Design review of the part built by this model. Coordinates are the model's own, in mm. Round coordinates to 2 decimals unless told otherwise and drop trailing zeros. Write each loop counter-clockwise with the first axis right and the second up, starting at its lowest first coordinate (ties: lowest second). Pieces come first, ordered by that corner, then holes. Notation, with made-up numbers: (26.5, 57) - (31.5, 57) arc R32 cw to (31.5, 84) - close; hole circle Ø8 at (47.5, 49). An arc over 180 degrees is marked (long way). Use one line per item in the form item = value.
```python
from build123d import *

# Parameters (mm, degrees)
F1_DEPTH = 1.5
F2_R     = 42.5
F3_DEPTH = 1.501
F4_R     = 10
F5_R     = 20
F7_D     = 6


with BuildPart() as f1:
    # F0 (on Top) → F1 (new body)
    with BuildSketch(Plane.XY):
        with BuildLine():
            Line((0, 36.5856099731), (0, 196.5856099731))
            ThreePointArc((0, 196.5856099731), (-307.3351576975, 315.2560594706), (-635, 349.5099039223))
            Line((-635, 349.5099039223), (-621.0269461922, 189.7971680702))
            Line((-621.0269461922, 189.7971680702), (-361.6779078132, 171.4103170113))
            Line((-361.6779078132, 171.4103170113), (-225.8692382849, 137.4102393502))
            Line((-225.8692382849, 137.4102393502), (0, 36.5856099731))
        make_face()
    extrude(amount=F1_DEPTH)

    # F2 (on face) → F3 (cut, through all)
    with BuildSketch(Plane.XY.offset(1.5)):
        with Locations((-275.0559937421, 229.17509395)):
            Circle(F2_R)
        with Locations((-165, 190)):
            Circle(F2_R)
        with Locations((-65, 145)):
            Circle(F2_R)
    extrude(amount=-F3_DEPTH, mode=Mode.SUBTRACT)

    # F4
    f4_edges = [f1.edges().sort_by_distance(p)[0] for p in [
        (0, 196.58561, 0.75),
        (-635, 349.509904, 0.75),
        (-621.026946, 189.797168, 0.75),
        (0, 36.58561, 0.75),
    ]]
    fillet(f4_edges, radius=F4_R)

    # F5
    f5_edges = [f1.edges().sort_by_distance(p)[0] for p in [
        (-361.677908, 171.410317, 0.75),
        (-225.869238, 137.410239, 0.75),
    ]]
    fillet(f5_edges, radius=F5_R)

    # F7 (through all)
    with Locations(Plane.XY.offset(1.5)):
        with Locations((-624.1092854766, 339.7655997622), (-611.8086529213, 199.1687262985), (-411.8395238612, 325.6409079413), (-374.0631195885, 182.3134808013), (-205.1081070963, 275.4405101573), (-209.8076952351, 141.1916790514), (-10, 190.6420127613), (-10, 52.0005303507)):
            Hole(F7_D / 2)


solid = f1.part
```
Q1. We need section A-A on y = 125. Write out the cut boundary in (x, z).
Calculated:
outline = (-198.07, 0) - (-102.5, 0) - (-102.5, 1.5) - (-198.07, 1.5) - close; (-27.5, 0) - (0, 0) - (0, 1.5) - (-27.5, 1.5) - close
Q2. We need section D-D on x = -542. Write out the cut boundary in (y, z).
Calculated:
outline = (184.19, 0) - (348.65, 0) - (348.65, 1.5) - (184.19, 1.5) - close
Q3. We need section B-B on x = -170.5. Write out the cut boundary in (y, z), then the cut area to 3 significant figures.
Calculated:
outline = (112.69, 0) - (147.86, 0) - (147.86, 1.5) - (112.69, 1.5) - close; (232.14, 0) - (273.9, 0) - (273.9, 1.5) - (232.14, 1.5) - close
area = 115 mm2
Q4. To check wall thickness, follow line 1 along X through (y, z) = (200, 1.1); line 2 along Y through (x, z) = (-10, 1.2); line 3 along Y through (x, z) = (-244, 1.35). State the ranges of each line that lie inside material, in increasing order. Write a range as from..to.
Calculated:
line_1 = -621.92..-614.69, -608.93..-305.96, -244.15..-206.31, -123.69..-6.28
line_2 = 42..49, 55..187.64, 193.64..202
line_3 = 141.95..200.16, 258.19..298.23
Q5. We need section C-C on z = 0.65. State how many separate pieces and enclosed holes the cut face has, then the cut area to 3 significant figures.
Calculated:
separate_pieces = 1
enclosed_holes = 11
area = 83,800 mm2
Q6. Draft analysis for pull direction Y (two halves, no side actions). For faces 1 (the cylindrical face through (-300.66, 313.63, 0.74)), 2 (the cylindrical face through (-317.515, 231.044, 0.76)), 3 (the flat face through (-120.65, 90.44, 0.74)), state which applies: released by +Y, released by -Y, zero draft, split by the parting line, or undercut.
Calculated:
face_1 = released by +Y
face_2 = undercut
face_3 = released by -Y
Q7. For P1, Ø1, axis at x = -435.5, y = 312, coming from the -Z side, flat-tipped, find the tip position at first contact; note if it passes through.
Calculated:
P1 = 0
